Verification items for the finished model (mm, model axes). A direction names the side the tool comes from. Coordinates: 2 decimals unless noted, no trailing zeros. Order: outer loops, then holes, each group sorted by start corner. A loop starts at its lowest first (then second) coordinate and runs counter-clockwise, first axis right, second up. Notation, with made-up numbers: M -9.75,63.25 L 17.25,63.25 A12 cw 17.25,74.25 Z; hole C -7,-28.75 d8. An arc over 180 degrees is marked long. Return JSON: item names as keys, results as strings. Group by question number.
Q1. Thickness scan on probe 1 along X at (y, z) = (-0.5, 50); probe 2 along Y at (x, z) = (-11.5, 28.5); probe 3 along Y at (x, z) = (-84, 47.5). Record the ranges inside material, lowest first.
Q2. Access from +Z, -Z, +X, -X, +Y, -Y to the whole of each face (thin tool, end or side, straight path). Record for faces 5 (the face through (-14, 11.137, 29)), 6 (the face through (-16, 12.137, 29)).
Q3. Section check B-B, the plane y = -3. Enter the section's corners in (x, z).
Q4. Section check A-A, the plane x = -34. Enter the section's corners in (y, z), then the cut area to 3 significant figures.
Q5. Section check C-C, the plane z = 46.5. Enter the section's corners in (x, y), then the cut area to 3 significant figures.
Q6. Go/stop test with flat-tipped pins: pin 1 Ø1.5 at (x, y) = (-5.5, 9.5) entering from +Z; pin 2 Ø5 at (x, y) = (-23.5, -12) entering from -Z; pin 3 Ø1.5 at (y, z) = (-7, 36) entering from -X; pin 4 Ø1 at (y, z) = (-5.5, 18.5) entering from -X. Record where each tip stops, or that it passes through.
Q7. Mould release check, pull along X, two halves, no side actions. Record for faces 1 (the face through (66.34, -1.07, 28.59)), 2 (the face through (-16, -13.863, 29)), 3 (the face through (-14, -14.863, 29)), 4 (the face through (-95.656, -1.088, 28.594)): pulls with the +X half, pulls with the -X half, needs draft (parallel to the pull), parting line crosses it, or undercut.
from build123d import *

# Parameters (mm, degrees)
BOSS_EXTRUDE1_DEPTH = 58


with BuildPart() as part:
    # Sketch1 → Boss-Extrude1 (new body)
    with BuildSketch(Plane.XY):
        with BuildLine():
            ThreePointArc((52.841370729, 12.137062925), (66.341370729, -1.362937075), (52.841370729, -14.862937075))
            Line((52.841370729, -14.862937075), (-83.158629271, -14.862937075))
            ThreePointArc((-83.158629271, -14.862937075), (-96.658629271, -1.362937075), (-83.158629271, 12.137062925))
            Line((-83.158629271, 12.137062925), (52.841370729, 12.137062925))
        make_face()
        with BuildLine():
            ThreePointArc((52.841370729, -13.862937075), (65.341370729, -1.362937075), (52.841370729, 11.137062925))
            Line((52.841370729, 11.137062925), (-83.158629271, 11.137062925))
            ThreePointArc((-83.158629271, 11.137062925), (-95.658629271, -1.362937075), (-83.158629271, -13.862937075))
            Line((-83.158629271, -13.862937075), (52.841370729, -13.862937075))
        make_face(mode=Mode.SUBTRACT)
    extrude(amount=BOSS_EXTRUDE1_DEPTH)


solid = part.part
Numbers:
{
 "1": {"probe 1": "x = -96.63 to -95.63, 65.31 to 66.31", "probe 2": "y = -14.86 to -13.86, 11.14 to 12.14", "probe 3": "y = -14.84 to -13.83, 11.11 to 12.11"},
 "2": {"face 5": "+Z, -Z", "face 6": "+Z, -Z, +X, -X, +Y"},
 "3": {"outline": "M -96.56,0 L -95.55,0 L -95.55,58 L -96.56,58 Z; M 65.23,0 L 66.24,0 L 66.24,58 L 65.23,58 Z"},
 "4": {"outline": "M -14.86,0 L -13.86,0 L -13.86,58 L -14.86,58 Z; M 11.14,0 L 12.14,0 L 12.14,58 L 11.14,58 Z", "area": "116 mm2"},
 "5": {"outline": "M -83.16,-14.86 L 52.84,-14.86 A13.5 ccw 52.84,12.14 L -83.16,12.14 A13.5 ccw Z; hole M -83.16,-13.86 L 52.84,-13.86 A12.5 ccw 52.84,11.14 L -83.16,11.14 A12.5 ccw Z", "area": "354 mm2"},
 "6": {"pin 1": "passes through", "pin 2": "stops at z = 0", "pin 3": "stops at x = -95.74", "pin 4": "stops at x = -96.16"},
 "7": {"face 1": "pulls with the +X half", "face 2": "undercut", "face 3": "needs draft", "face 4": "undercut"}
}
